Design review of the part built by this model. Coordinates are the model's own, in mm. A direction names the side the tool comes from. Coordinates: 2 decimals unless noted, no trailing zeros. Loops run counter-clockwise (first coordinate to the right, second up) from the corner with the lowest first, then second, coordinate; pieces in that order, holes last. Notation, with made-up numbers: M 15.25,-8.75 L 39.25,-8.75 A23 ccw 39.25,27.25 Z; hole C 32.25,22 d9. An arc over 180 degrees is marked long. Write item = value, one per line. Start each with the question number.
from build123d import *

# Parameters (mm, degrees)
SKETCH1_R           = 1.9
BOSS_EXTRUDE1_DEPTH = 6
SKETCH2_W           = 142.5
SKETCH2_H           = 5
SKETCH2_W_2         = 22.5
CUT_EXTRUDE1_DEPTH  = 98.812320287
SKETCH3_W           = 10
SKETCH3_H           = 5
BOSS_EXTRUDE2_DEPTH = 6


with BuildPart() as part:
    # Sketch1 → Boss-Extrude1 (new body)
    with BuildSketch(Plane.XY):
        with BuildLine():
            Line((-92.5, 5), (92.5, 5))
            ThreePointArc((92.5, 5), (97.5, 0), (92.5, -5))
            Line((92.5, -5), (-92.5, -5))
            ThreePointArc((-92.5, -5), (-97.5, 0), (-92.5, 5))
        make_face()
        with Locations((-92.5, 0)):
            Circle(SKETCH1_R, mode=Mode.SUBTRACT)
        with Locations((92.5, 0)):
            Circle(SKETCH1_R, mode=Mode.SUBTRACT)
        with Locations((60, 0)):
            Circle(SKETCH1_R, mode=Mode.SUBTRACT)
    extrude(amount=BOSS_EXTRUDE1_DEPTH)

    # Sketch2 → Cut-Extrude1 (cut, through all)
    with BuildSketch(Plane.XY.offset(6)):
        with Locations((-16.25, 0)):
            Rectangle(SKETCH2_W, SKETCH2_H)
        with Locations((76.25, 0)):
            Rectangle(SKETCH2_W_2, SKETCH2_H)
    extrude(amount=-CUT_EXTRUDE1_DEPTH, mode=Mode.SUBTRACT)

    # Sketch3 → Boss-Extrude2 (add, through all)
    with BuildSketch(Plane.XY.offset(6)):
        with Locations((-13.75, 0)):
            Rectangle(SKETCH3_W, SKETCH3_H)
    extrude(amount=-BOSS_EXTRUDE2_DEPTH)


solid = part.part
Q1. Add section B-B on z = 1.25. State the section outline as (x, y) points.
Q2. Clearance check with flat-ended pins moving along their axes: P1, Ø1, axis at x = -51.5, y = 1.5, coming from the -Z side; P2, Ø1.5, axis at y = 2, z = 4, coming from the -X side. State where each tip first meets the part, or that it passes through.
Q3. For faces 4 (the face through (97.5, 0.1, 3)), 5 (the face through (76, -2.5, 3)), list the 3-axis set-ups (+Z, -Z, +X, -X, +Y, -Y) from which the entire face can be reached by the end or side of a thin tool; tool diameter is ignored.
Q4. Mouldability with a two-part tool opening along X and no side actions: class faces 1 (the face through (-97.5, -0.1, 3)), 2 (the face through (55, 0, 3)), 3 (the face through (1, -5, 3)) as released by +X, released by -X, zero draft, split by the parting line, or undercut.
Q5. Add section A-A on x = -26.5. State the section outline as (y, z) points.
Q6. Add section C-C on x = 60. State the section outline as (y, z) points, plus the area to 3 significant figures.
Q7. To check wall thickness, follow line 1 (Y direction, x = 16, z = 3.7); line 2 (Y direction, x = -92.5, z = 3.75); line 3 (X direction, y = -2.25, z = 5.4). State the ranges of each line that lie inside material, in increasing order. Write a range as from..to.
Values follow:
q1.outline = M -92.5,-5 L 92.5,-5 A5 ccw 92.5,5 L -92.5,5 A5 ccw Z; hole C -92.5,0 d3.8; hole M -87.5,-2.5 L -18.75,-2.5 L -18.75,2.5 L -87.5,2.5 Z; hole M -8.75,-2.5 L 55,-2.5 L 55,2.5 L -8.75,2.5 Z; hole C 60,0 d3.8; hole M 65,-2.5 L 87.5,-2.5 L 87.5,2.5 L 65,2.5 Z; hole C 92.5,0 d3.8
q2.P1 = through
q2.P2 = -97.34
q3.face_4 = +Z, -Z, +X
q3.face_5 = +Z, -Z
q4.face_1 = released by -X
q4.face_2 = undercut
q4.face_3 = zero draft
q5.outline = M -5,0 L -2.5,0 L -2.5,6 L -5,6 Z; M 2.5,0 L 5,0 L 5,6 L 2.5,6 Z
q6.outline = M -5,0 L -1.9,0 L -1.9,6 L -5,6 Z; M 1.9,0 L 5,0 L 5,6 L 1.9,6 Z
q6.area = 37.2 mm2
q7.line_1 = -5..-2.5, 2.5..5
q7.line_2 = -5..-1.9, 1.9..5
q7.line_3 = -96.97..-87.5, -18.75..-8.75, 55..65, 87.5..96.97
